from build123d import *

# Parameters (mm, degrees)
SKETCH1_R           = 2.4892
BOSS_EXTRUDE1_DEPTH = 6.477
FILLET2_R           = 6.35
FILLET3_R           = 3.175


with BuildPart() as part:
    # Sketch1 → Boss-Extrude1 (new body)
    with BuildSketch(Plane.XY):
        Polygon((0, 0), (40.53078, 0), (421.903292844, 0), (421.903292844, -9.525), (447.303292844, -9.525), (447.303292844, 0), (584.2, 0), (584.2, 25.4), (40.530665192, 25.4), (40.530665192, 34.925), (15.130665192, 34.925), (15.130665192, 25.4), (0, 25.4), align=None)
        with Locations((577.85, 6.35)):
            Circle(SKETCH1_R, mode=Mode.SUBTRACT)
    extrude(amount=BOSS_EXTRUDE1_DEPTH)

    # Fillet2
    fillet2_edges = [part.edges().sort_by_distance(p)[0] for p in [
        (0, 0, 3.2385),
        (0, 25.4, 3.2385),
        (584.2, 25.4, 3.2385),
        (584.2, 0, 3.2385),
    ]]
    fillet(fillet2_edges, radius=FILLET2_R)


with BuildPart() as body_2:
    # Mirror2: mirrored copy
    add(part.part.mirror(Plane.XY))

    # Fillet3
    fillet3_edges = [body_2.edges().sort_by_distance(p)[0] for p in [
        (447.303292844, -9.525, -3.2385),
        (421.903292844, -9.525, -3.2385),
        (421.903292844, 0, -3.2385),
        (15.130665192, 25.4, -3.2385),
        (15.130665192, 34.925, -3.2385),
        (40.530665192, 34.925, -3.2385),
        (40.530665192, 25.4, -3.2385),
        (447.303292844, 0, -3.2385),
    ]]
    fillet(fillet3_edges, radius=FILLET3_R)


solid = body_2.part
Geometry: final body of the model. Coordinates: model frame, mm. Give positions to 0.01 mm unless a question says otherwise; leave off trailing zeros. Loops run counter-clockwise (first coordinate to the right, second up) from the corner with the lowest first, then second, coordinate; pieces in that order, holes last. Notation, with made-up numbers: M 50,-9.5 L 68,-9.5 A21 cw 68,25.5 Z; hole C 16.25,37 d1. An arc over 180 degrees is marked long. Put each result on its own line as item: value.
1) Cut plane C-C, the plane x = 431. Return the cut outline in (y, z) (3 decimals).
Computed values:
outline: M -9.525,-6.477 L 25.4,-6.477 L 25.4,0 L -9.525,0 Z
2) Cut plane B-B, the plane x = 536.5. Return the cut outline in (y, z).
Computed values:
outline: M 0,-6.48 L 25.4,-6.48 L 25.4,0 L 0,0 Z
3) Material intervals for L1, parallel to Y at x = 577.85, z = -2.5; L2, parallel to Y at x = 323.5, z = -6; L3, parallel to X at y = 5, z = -4.25, sorted ascending. Write a range as from..to.
Computed values:
L1: y = 0..3.86, 8.84..25.4
L2: y = 0..25.4
L3: x = 0.15..575.76, 579.94..584.05
4) Cut plane A-A, the plane z = -2.25. Return the cut outline in (x, y) (3 decimals), plus the area to 3 significant figures.
Computed values:
outline: M 0,6.35 A6.35 ccw 6.35,0 L 418.728,0 A3.175 cw 421.903,-3.175 L 421.903,-6.35 A3.175 ccw 425.078,-9.525 L 444.128,-9.525 A3.175 ccw 447.303,-6.35 L 447.303,-3.175 A3.175 cw 450.478,0 L 577.85,0 A6.35 ccw 584.2,6.35 L 584.2,19.05 A6.35 ccw 577.85,25.4 L 43.706,25.4 A3.175 cw 40.531,28.575 L 40.531,31.75 A3.175 ccw 37.356,34.925 L 18.306,34.925 A3.175 ccw 15.131,31.75 L 15.131,28.575 A3.175 cw 11.956,25.4 L 6.35,25.4 A6.35 ccw 0,19.05 Z; hole C 577.85,6.35 d4.978
area: 15,300 mm^2
5) First-contact query: P1, Ø1, axis at y = 30.5, z = -2.5, coming from the -X side; P2, Ø1.6, axis at y = -5, z = -2.5, coming from the -X side; P3, Ø1, axis at y = 30.5, z = -3, coming from the +X side; P4, Ø10, axis at x = 307, y = 30, coming from the +Z side. Flat tips, straight axial feed; report the tip coordinate or a pass-through.
Computed values:
P1: stops at x = 15.13
P2: stops at x = 421.9
P3: stops at x = 40.53
P4: stops at z = 0
